from build123d import *

# Parameters (mm, degrees)
SKETCH1_W            = 65
SKETCH1_H            = 48
BOSS_EXTRUDE1_DEPTH  = 2
M3_CLEARANCE_HOLE1_D = 4
SKETCH5_W            = 8
SKETCH5_H            = 8
BOSS_EXTRUDE2_DEPTH  = 6
CUT_EXTRUDE1_DEPTH   = 48.271281194
FILLET4_R            = 3


with BuildPart() as part:
    # Sketch1 → Boss-Extrude1 (new body)
    with BuildSketch(Plane.XY):
        with Locations((4.50867052, -4.791184971)):
            Rectangle(SKETCH1_W, SKETCH1_H)
    extrude(amount=BOSS_EXTRUDE1_DEPTH)

    # M3 Clearance Hole1 (through all)
    with Locations(Plane.XY.offset(2)):
        with Locations((4.50867052, 4.208815029), (4.50867052, -5.791184971)):
            Hole(M3_CLEARANCE_HOLE1_D / 2)

    # Sketch5 → Boss-Extrude2 (add)
    with BuildSketch(Plane.XY.offset(2)):
        with Locations((4.50867052, -24.791184971)):
            Rectangle(SKETCH5_W, SKETCH5_H)
    extrude(amount=BOSS_EXTRUDE2_DEPTH)

    # Sketch6 → Cut-Extrude1 (cut, through all)
    with BuildSketch(Plane.XY.offset(2)):
        Polygon((-27.99132948, -28.791184971), (0.50867052, -28.791184971), (0.50867052, -20.791184971), (0.50867052, 8.208815029), (8.50867052, 8.208815029), (8.50867052, -20.791184971), (8.50867052, -28.791184971), (37.00867052, -28.791184971), (37.00867052, 19.208815029), (-27.99132948, 19.208815029), align=None)
    extrude(amount=-CUT_EXTRUDE1_DEPTH, mode=Mode.SUBTRACT)

    # Fillet4
    fillet4_edges = [part.edges().sort_by_distance(p)[0] for p in [
        (8.50867052, -28.791184971, 4),
        (4.50867052, -20.791184971, 2),
        (4.50867052, -20.791184971, 8),
        (0.50867052, 8.208815029, 1),
        (8.50867052, 8.208815029, 1),
        (0.50867052, -28.791184971, 4),
    ]]
    fillet(fillet4_edges, radius=FILLET4_R - 0.0001)  # a hair under: the kernel refuses the full size


solid = part.part
Verification items for the finished model (mm, model axes). Coordinates: 2 decimals unless noted, no trailing zeros. Loops run counter-clockwise (first coordinate to the right, second up) from the corner with the lowest first, then second, coordinate; pieces in that order, holes last. Notation, with made-up numbers: (55, 45.5) -> (59, 45.5) arc R24 cw to (59, 57.5) -> close; hole circle Ø7 at (67.5, 89). An arc over 180 degrees is marked (long way). Answer as a JSON object with one key per item and string values. Group by question number.
Item 1: Sectioned sample at A-A on x = 4.25. State how many separate pieces and enclosed holes the cut face has, plus the area to 3 significant figures.
Item 2: Sectioned sample at C-C on y = -17. Record the boundary of the cut face in (x, z).
Item 3: Mould release check, pull along X, two halves, no side actions. Record for faces 1 (the flat face through (2.7, -4.6, 2)), 2 (the cylindrical face through (1.41, 7.35, 0.99)), 3 (the cylindrical face through (4.942, -7.744, 0.986)), 4 (the flat face through (8.509, -14.8, 1.6)): +X half, -X half, draft (parallel to the pull), parting line (faces both ways), or undercut.
Item 4: Sectioned sample at B-B on z = 3. Record the boundary of the cut face in (x, y).
Item 5: Scan lines: probe 1 along Y at (x, z) = (6.25, 1.25); probe 2 along Z at (x, y) = (8, -15); probe 3 along Y at (x, z) = (8.25, 2.75). Record each from-to range of solid material in increasing order.
Item 6: Depth check by flat-ended pin: pin 1 (2.5 mm diameter, centred on x = 5, y = -8, fed in from +Z); pin 2 (2 mm diameter, centred on x = 7, z = 4.5, fed in from +Y). Enter the tip coordinate at first touch or a pass-through.
Evaluation:
{
 "1": {"separate pieces": "3", "enclosed holes": "0", "area": "106 mm²"},
 "2": {"outline": "(0.51, 0) -> (8.51, 0) -> (8.51, 2) -> (0.51, 2) -> close"},
 "3": {"face 1": "draft", "face 2": "-X half", "face 3": "undercut", "face 4": "+X half"},
 "4": {"outline": "(0.51, -25.79) arc R3 ccw to (3.51, -28.79) -> (5.51, -28.79) arc R3 ccw to (8.51, -25.79) -> (8.51, -20.03) -> (0.51, -20.03) -> close"},
 "5": {"probe 1": "y = -28.7 to -6.77, -4.81 to 3.23, 5.19 to 8.12", "probe 2": "z = 0 to 2", "probe 3": "y = -27.01 to -19.78"},
 "6": {"pin 1": "stops at z = 2", "pin 2": "stops at y = -20.39"}
}
